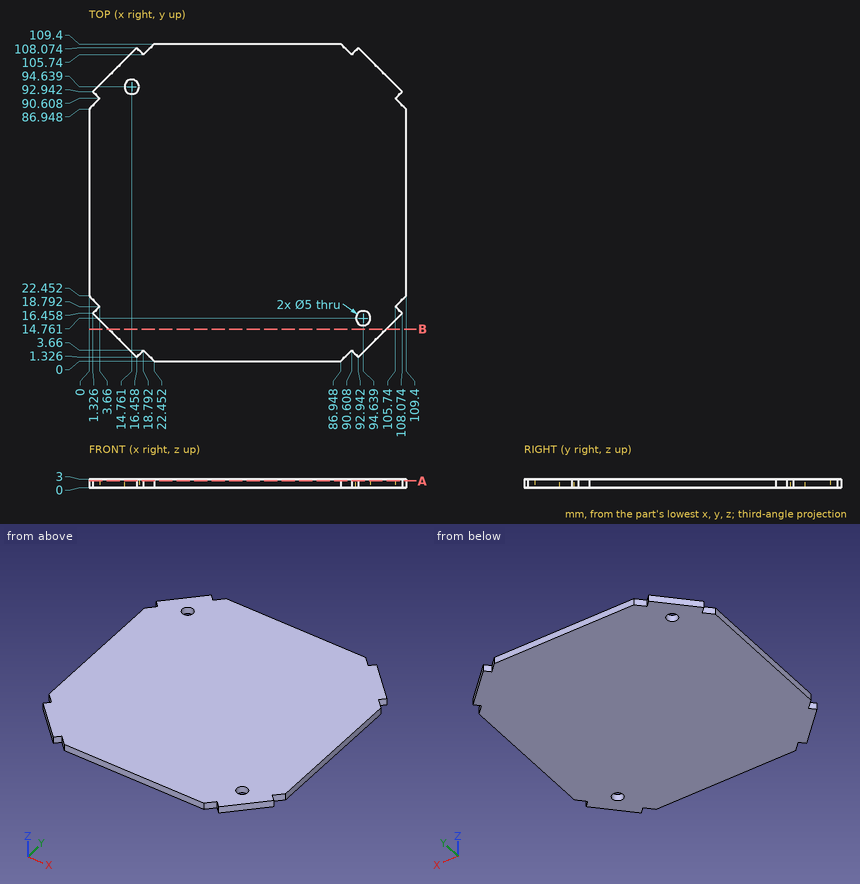
The drawing under review shows one solid part. Ordinate dimensions are in mm from its lowest x, y, z. Round coordinates to 2 decimals unless told otherwise and drop trailing zeros. Order: outer loops, then holes, each group sorted by start corner. A loop starts at its lowest first (then second) coordinate and runs counter-clockwise, first axis right, second up. Notation, with made-up numbers: (-35.75, 80) - (-2.75, 80) arc R19 cw to (-2.75, 88) - close; hole circle Ø7 at (9, 69). An arc over 180 degrees is marked (long way). Return JSON: item names as keys, results as strings.
Q1. Consider section B-B on y = 11. Write out the cut boundary in (x, z) (1 decimal).
Computed values:
{"outline": "(6.8, 0) - (102.6, 0) - (102.6, 3) - (6.8, 3) - close"}
Q2. For pin 1 Ø4 at (x, y) = (94.64, 14.76) entering from -Z, flat-tipped, find the tip position at first contact; note if it passes through.
Computed values:
{"pin 1": "passes through"}
Q3. Wall thickness on L1, parallel to Y at x = 96.5, z = 1.25 (1 decimal); L2, parallel to X at y = 96, z = 0.2 (1 decimal); L3, parallel to Y at x = 19, z = 2.6: over which ranges is each line inside the solid? List them lowest first. Write a range as [from, to].
Computed values:
{"L1": "y = [4.9, 13.1], [16.4, 104.5]", "L2": "x = [4.4, 12.7], [16.9, 105]", "L3": "y = [3.45, 105.95]"}
Q4. Consider section A-A on z = 2.35. Write out the cut boundary in (x, y).
Computed values:
{"outline": "(0, 22.45) - (3.66, 18.79) - (1.33, 16.46) - (16.46, 1.33) - (18.79, 3.66) - (22.45, 0) - (86.95, 0) - (90.61, 3.66) - (92.94, 1.33) - (108.07, 16.46) - (105.74, 18.79) - (109.4, 22.45) - (109.4, 86.95) - (105.74, 90.61) - (108.07, 92.94) - (92.94, 108.07) - (90.61, 105.74) - (86.95, 109.4) - (22.45, 109.4) - (18.79, 105.74) - (16.46, 108.07) - (1.33, 92.94) - (3.66, 90.61) - (0, 86.95) - close; hole circle Ø5 at (14.76, 94.64); hole circle Ø5 at (94.64, 14.76)"}
